from build123d import *

# Parameters (mm, degrees)
SKETCH2_OUTSIDE_W        = 55.898
SKETCH2_OUTSIDE_H        = 55.898
SKETCH2_OUTSIDE_R        = 12.5
CUT_EXTRUDE_DEPTH        = 4.346553008
PATTERN_CIRCULAR_4_COUNT = 17
EXTRUDE_1_DEPTH          = 1.25


with BuildPart() as part:
    # Sketch1 → Base-Extrude (revolve)
    with BuildSketch(Plane.YZ):
        Polygon((0, -3.346553008), (-16, -3.346553008), (-21, -1.143921767), (-20.496072436, 0), (-16, -2.096553008), (0, -2.096553008), align=None)
    revolve(axis=Axis((0, 0, 5.823648763), (0, 0, -1)))

    # Sketch2 outside → Cut-Extrude (cut, through all)
    with BuildSketch(Plane(origin=(-2.40435344, 1.003568156, -3.346553008), x_dir=(-1, 0, 0), z_dir=(0, 0, -1))):
        with Locations((-2.404, -1.004)):
            Rectangle(SKETCH2_OUTSIDE_W, SKETCH2_OUTSIDE_H)
        with BuildLine():
            Line((-15.182466724, 8.625545038), (-19.50954274, 11.178898713))
            ThreePointArc((-19.50954274, 11.178898713), (-20.590886919, 9.496431844), (-21.507273879, 7.718726879))
            Line((-21.507273879, 7.718726879), (-17.132466724, 5.248045963))
            ThreePointArc((-17.132466724, 5.248045963), (11.452053021, -9.003568156), (-15.182466724, 8.625545038))
        make_face(mode=Mode.SUBTRACT)
        with Locations((-2.40435344, -1.003568156)):
            Circle(SKETCH2_OUTSIDE_R)
    extrude(amount=-CUT_EXTRUDE_DEPTH, mode=Mode.SUBTRACT)


with BuildPart() as pattern_circular_4_1:
    # Pattern Circular 4: pattern copy
    add(part.part.rotate(Axis((0, 0, 0), (0, 0, 1)), 1 * 360 / PATTERN_CIRCULAR_4_COUNT))


with BuildPart() as pattern_circular_4_2:
    # Pattern Circular 4: pattern copy
    add(part.part.rotate(Axis((0, 0, 0), (0, 0, 1)), 2 * 360 / PATTERN_CIRCULAR_4_COUNT))


with BuildPart() as pattern_circular_4_3:
    # Pattern Circular 4: pattern copy
    add(part.part.rotate(Axis((0, 0, 0), (0, 0, 1)), 3 * 360 / PATTERN_CIRCULAR_4_COUNT))


with BuildPart() as pattern_circular_4_4:
    # Pattern Circular 4: pattern copy
    add(part.part.rotate(Axis((0, 0, 0), (0, 0, 1)), 4 * 360 / PATTERN_CIRCULAR_4_COUNT))


with BuildPart() as pattern_circular_4_5:
    # Pattern Circular 4: pattern copy
    add(part.part.rotate(Axis((0, 0, 0), (0, 0, 1)), 5 * 360 / PATTERN_CIRCULAR_4_COUNT))


with BuildPart() as pattern_circular_4_6:
    # Pattern Circular 4: pattern copy
    add(part.part.rotate(Axis((0, 0, 0), (0, 0, 1)), 6 * 360 / PATTERN_CIRCULAR_4_COUNT))


with BuildPart() as pattern_circular_4_7:
    # Pattern Circular 4: pattern copy
    add(part.part.rotate(Axis((0, 0, 0), (0, 0, 1)), 7 * 360 / PATTERN_CIRCULAR_4_COUNT))


with BuildPart() as pattern_circular_4_8:
    # Pattern Circular 4: pattern copy
    add(part.part.rotate(Axis((0, 0, 0), (0, 0, 1)), 8 * 360 / PATTERN_CIRCULAR_4_COUNT))


with BuildPart() as pattern_circular_4_9:
    # Pattern Circular 4: pattern copy
    add(part.part.rotate(Axis((0, 0, 0), (0, 0, 1)), 9 * 360 / PATTERN_CIRCULAR_4_COUNT))


with BuildPart() as pattern_circular_4_10:
    # Pattern Circular 4: pattern copy
    add(part.part.rotate(Axis((0, 0, 0), (0, 0, 1)), 10 * 360 / PATTERN_CIRCULAR_4_COUNT))


with BuildPart() as pattern_circular_4_11:
    # Pattern Circular 4: pattern copy
    add(part.part.rotate(Axis((0, 0, 0), (0, 0, 1)), 11 * 360 / PATTERN_CIRCULAR_4_COUNT))


with BuildPart() as pattern_circular_4_12:
    # Pattern Circular 4: pattern copy
    add(part.part.rotate(Axis((0, 0, 0), (0, 0, 1)), 12 * 360 / PATTERN_CIRCULAR_4_COUNT))


with BuildPart() as pattern_circular_4_13:
    # Pattern Circular 4: pattern copy
    add(part.part.rotate(Axis((0, 0, 0), (0, 0, 1)), 13 * 360 / PATTERN_CIRCULAR_4_COUNT))


with BuildPart() as pattern_circular_4_14:
    # Pattern Circular 4: pattern copy
    add(part.part.rotate(Axis((0, 0, 0), (0, 0, 1)), 14 * 360 / PATTERN_CIRCULAR_4_COUNT))


with BuildPart() as pattern_circular_4_15:
    # Pattern Circular 4: pattern copy
    add(part.part.rotate(Axis((0, 0, 0), (0, 0, 1)), 15 * 360 / PATTERN_CIRCULAR_4_COUNT))


with BuildPart() as pattern_circular_4_16:
    # Pattern Circular 4: pattern copy
    add(part.part.rotate(Axis((0, 0, 0), (0, 0, 1)), 16 * 360 / PATTERN_CIRCULAR_4_COUNT))


with BuildPart() as part_1:
    add(part.part)

    add(pattern_circular_4_1.part)  # Extrude 1 merges Pattern Circular 4_1

    add(pattern_circular_4_2.part)  # Extrude 1 merges Pattern Circular 4_2

    add(pattern_circular_4_3.part)  # Extrude 1 merges Pattern Circular 4_3

    add(pattern_circular_4_4.part)  # Extrude 1 merges Pattern Circular 4_4

    add(pattern_circular_4_5.part)  # Extrude 1 merges Pattern Circular 4_5

    add(pattern_circular_4_6.part)  # Extrude 1 merges Pattern Circular 4_6

    add(pattern_circular_4_7.part)  # Extrude 1 merges Pattern Circular 4_7

    add(pattern_circular_4_8.part)  # Extrude 1 merges Pattern Circular 4_8

    add(pattern_circular_4_9.part)  # Extrude 1 merges Pattern Circular 4_9

    add(pattern_circular_4_10.part)  # Extrude 1 merges Pattern Circular 4_10

    add(pattern_circular_4_11.part)  # Extrude 1 merges Pattern Circular 4_11

    add(pattern_circular_4_12.part)  # Extrude 1 merges Pattern Circular 4_12

    add(pattern_circular_4_13.part)  # Extrude 1 merges Pattern Circular 4_13

    add(pattern_circular_4_14.part)  # Extrude 1 merges Pattern Circular 4_14

    add(pattern_circular_4_15.part)  # Extrude 1 merges Pattern Circular 4_15

    add(pattern_circular_4_16.part)  # Extrude 1 merges Pattern Circular 4_16
    # Sketch 2 → Extrude 1 (add)
    with BuildSketch(Plane.XY.offset(-2.096553008)):
        with BuildLine():
            Line((1.848868807, 10.633987217), (1.741294281, 12.378121595))
            ThreePointArc((1.741294281, 12.378121595), (-0.769511327, 12.476291609), (-3.249222363, 12.070317065))
            Line((-3.249222363, 12.070317065), (-3.141647836, 10.326182686))
            Line((-3.141647836, 10.326182686), (1.848868807, 10.633987217))
        make_face()
    extrude(amount=-EXTRUDE_1_DEPTH)


solid = part_1.part
Design review of the part built by this model. Coordinates are the model's own, in mm. A direction names the side the tool comes from. Coordinates: 2 decimals unless noted, no trailing zeros. Order: outer loops, then holes, each group sorted by start corner. A loop starts at its lowest first (then second) coordinate and runs counter-clockwise, first axis right, second up.
Item 1: For line 1 (Z direction, x = 11, y = 9); line 2 (X direction, y = 0, z = -2.7); line 3 (X direction, y = 0, z = -2.5), list the stretches that pass through material, from the lowest coordinate up.
Item 2: Take a section at A-A, the plane y = 0. Write out the cut boundary in (x, z).
Item 3: For faces 5 (the conical face through (10.55, -14.85, -1.063)), 6 (the flat face through (13.09, 13.12, -1.7)), 7 (the flat face through (-11.86, 14.25, -1.7)), list the 3-axis set-ups (+Z, -Z, +X, -X, +Y, -Y) from which the entire face can be reached by the end or side of a thin tool; tool diameter is ignored.
Item 4: The part is to be moulded in two halves that separate along X. For faces 1 (the flat face through (-4.224, -18.046, -1.697)), 2 (the conical face through (20.495, 3.21, -0.564)), 3 (the flat face through (-3.1, 18.2, -1.7)), 4 (the conical face through (-15.735, -13.518, -0.564)), say which applies: pulls with the +X half, pulls with the -X half, needs draft (parallel to the pull), parting line crosses it, or undercut.
Item 5: For pin 1 Ø1.5 at (x, z) = (5, -1) entering from -Y; pin 2 Ø9.5 at (x, y) = (-7, -4) entering from +Z; pin 3 Ø2 at (x, y) = (-11, 10.5) entering from +Z, all flat-tipped, find the tip position at first contact; note any pin that passes through.
The answers:
1. line 1: z = -3.35 to -2.1
1. line 2: x = -17.47 to -12.5, 12.5 to 16
1. line 3: x = -17.92 to -12.5, 12.5 to 16
2. outline: (-21, -1.14) - (-16, -3.35) - (-12.5, -3.35) - (-12.5, -2.1) - (-16, -2.1) - (-20.5, 0) - close; (12.5, -3.35) - (16, -3.35) - (16, -2.1) - (12.5, -2.1) - close
3. face 5: +Z
3. face 6: +Z, -Z, +X
3. face 7: +Z, -Z, +Y
4. face 1: undercut
4. face 2: pulls with the +X half
4. face 3: undercut
4. face 4: pulls with the -X half
5. pin 1: stops at y = -20.56
5. pin 2: stops at z = -2.1
5. pin 3: stops at z = -2
